Input: part model. Units: mm. Frame: model coordinates. A direction names the side the tool comes from. Round coordinates to 2 decimals unless told otherwise and drop trailing zeros. Write each loop counter-clockwise with the first axis right and the second up, starting at its lowest first coordinate (ties: lowest second). Pieces come first, ordered by that corner, then holes. Notation, with made-up numbers: (15, -7.5) -> (53, -7.5) arc R19 ccw to (53, 3.5) -> close; hole circle Ø5 at (6.5, 27.25). An arc over 180 degrees is marked (long way). Use CSV: the item, a comma, the result in double quotes.
```python
from build123d import *

# Parameters (mm, degrees)
SKETCH1_W           = 6
SKETCH1_H           = 6
BOSS_EXTRUDE1_DEPTH = 5
CUT_EXTRUDE9_DEPTH  = 23.5
CUT_EXTRUDE10_DEPTH = 3


with BuildPart() as part:
    # Sketch1 → Boss-Extrude1 (new body)
    with BuildSketch(Plane(origin=(0, 0, 0), x_dir=(1, 0, 0), z_dir=(0, 1, 0))):
        Rectangle(SKETCH1_W, SKETCH1_H)
    extrude(amount=BOSS_EXTRUDE1_DEPTH)

    # Sketch12 → Cut-Extrude9 (cut)
    with BuildSketch(Plane.ZY.offset(3)):
        Polygon((-3, 0), (3, 5), (-3, 5), align=None)
    extrude(amount=-CUT_EXTRUDE9_DEPTH, mode=Mode.SUBTRACT)

    # Sketch13 → Cut-Extrude10 (cut)
    with BuildSketch(Plane.ZY.offset(3)):
        Polygon((3, 5), (0, 2.5), (3, 2.5), align=None)
    extrude(amount=-CUT_EXTRUDE10_DEPTH, mode=Mode.SUBTRACT)


solid = part.part
```
Item 1: Set-up query: faces 1 (the face through (0, 3, 2)), 2 (the face through (0, 0, 0)). Return all of +Z, -Z, +X, -X, +Y, -Y with unobstructed straight access to the full face (end or side cutting, diameter ignored); none if empty.
Worked answers:
face 1,"+Z, -Z, -X, +Y"
face 2,"+Z, -Z, +X, -X, -Y"
Item 2: Section query D-D on z = -1.8. Return the cut outline in (x, y).
Worked answers:
outline,"(-3, 0) -> (3, 0) -> (3, 1) -> (-3, 1) -> close"
Item 3: First-contact query: pin 1 Ø0.9 at (x, z) = (-1, 2) entering from +Y; pin 2 Ø0.8 at (y, z) = (3.5, 1) entering from -X. Flat tips, straight axial feed; report the tip coordinate or a pass-through.
Worked answers:
pin 1,"stops at y = 2.5"
pin 2,"stops at x = 0"
Item 4: Section query C-C on x = 1.55. Return the cut outline in (y, z), plus the area to 3 significant figures.
Worked answers:
outline,"(0, -3) -> (5, 3) -> (0, 3) -> close"
area,"15.0 mm²"
Item 5: Line query: line 1 (X direction, y = 3.2, z = 1.65); line 2 (Y direction, x = -2.7, z = 0.05); line 3 (Y direction, x = 0.2, z = -2.3). Output: solid intervals per line, ascending.
Worked answers:
line 1,"x = 0 to 3"
line 2,"y = 0 to 2.5"
line 3,"y = 0 to 0.58"
Item 6: Section query A-A on z = 0.6. Return the cut outline in (x, y).
Worked answers:
outline,"(-3, 0) -> (3, 0) -> (3, 3) -> (0, 3) -> (0, 2.5) -> (-3, 2.5) -> close"
Item 7: Section query B-B on y = 3.55. Return the cut outline in (x, z), plus the area to 3 significant figures.
Worked answers:
outline,"(0, 1.26) -> (3, 1.26) -> (3, 3) -> (0, 3) -> close"
area,"5.22 mm²"
